Part model, mm, in its own coordinate system. Round coordinates to 2 decimals unless told otherwise and drop trailing zeros. Loops run counter-clockwise (first coordinate to the right, second up) from the corner with the lowest first, then second, coordinate; pieces in that order, holes last. Notation, with made-up numbers: (26.25, -40) - (70.25, -40) arc R28 cw to (70.25, -15) - close; hole circle Ø1 at (7, 27). An arc over 180 degrees is marked (long way). Write each question's results on one line, items separated by ' | '. Start each with the question number.
(1) Cut at B-B, the plane z = 5. List the corners of the cut face in (x, y), then the cut area to 3 significant figures.
(2) Mould opens along X. For faces 1 (the face through (0, 41, 0)), 2 (the face through (0.273, 42.282, 7.918)), 3 (the face through (-14.985, 42.479, 0.66)) say: released by +X, released by -X, zero draft, split by the parting line, or undercut.
(3) Cut at A-A, the plane x = 0. List the corners of the cut face in (y, z).
(4) Drill centre lines: L1, parallel to Z at x = 0, y = 42.8; L2, parallel to Z at x = 1.75, y = 41.75; L3, parallel to X at y = 43.9, z = 8. Where is each one in solid material? Low to high.
(5) Cut at C-C, the plane y = 41.7. List the corners of the cut face in (x, z), then the cut area to 3 significant figures.
(6) Cut at D-D, the plane z = -10. List the corners of the cut face in (x, y).
from build123d import *

# Parameters (mm, degrees)
SKETCH_1_R                  = 15
EXTRUDE_1_DEPTH             = 3
HOLE_WIZARD_M41_D           = 4.2
HOLE_WIZARD_M41_CSINK_D     = 5
HOLE_WIZARD_M41_CSINK_ANGLE = 90


with BuildPart() as part:
    # Эскиз1 → Бобышка-Вытянуть1 (new body)
    with BuildSketch(Plane.XZ.offset(-41)):
        Circle(SKETCH_1_R)
    extrude(amount=-EXTRUDE_1_DEPTH)

    # Сверло под метчик  спиральное M41 (through all)
    with Locations(Plane(origin=(0, 44, 0), x_dir=(1, 0, 0), z_dir=(0, 1, 0))):
        with Locations((-8.660254038, 5), (0, 10), (8.660254038, 5), (8.660254038, -5), (0, -10), (-8.660254038, -5)):
            CounterSinkHole(HOLE_WIZARD_M41_D / 2, HOLE_WIZARD_M41_CSINK_D / 2, counter_sink_angle=HOLE_WIZARD_M41_CSINK_ANGLE)


solid = part.part
A:
1) outline: (-14.14, 41) - (-10.76, 41) - (-10.76, 43.6) - (-11.16, 44) - (-14.14, 44) - close; (-6.56, 41) - (6.56, 41) - (6.56, 43.6) - (6.16, 44) - (-6.16, 44) - (-6.56, 43.6) - close; (10.76, 41) - (14.14, 41) - (14.14, 44) - (11.16, 44) - (10.76, 43.6) - close | area: 59.3 mm2
2) face 1: zero draft | face 2: undercut | face 3: split by the parting line
3) outline: (41, -15) - (44, -15) - (44, -12.5) - (43.6, -12.1) - (41, -12.1) - close; (41, -7.9) - (43.6, -7.9) - (44, -7.5) - (44, 7.5) - (43.6, 7.9) - (41, 7.9) - close; (41, 12.1) - (43.6, 12.1) - (44, 12.5) - (44, 15) - (41, 15) - close
4) L1: -15 to -12.1, -7.9 to 7.9, 12.1 to 15 | L2: -14.9 to -11.16, -8.84 to 8.84, 11.16 to 14.9 | L3: -12.69 to -1.33, 1.33 to 12.69
5) outline: circle Ø30 at (0, 0); hole circle Ø4.2 at (-8.66, -5); hole circle Ø4.2 at (-8.66, 5); hole circle Ø4.2 at (0, -10); hole circle Ø4.2 at (0, 10); hole circle Ø4.2 at (8.66, -5); hole circle Ø4.2 at (8.66, 5) | area: 624 mm2
6) outline: (-11.18, 41) - (-2.1, 41) - (-2.1, 43.6) - (-2.5, 44) - (-11.18, 44) - close; (2.1, 41) - (11.18, 41) - (11.18, 44) - (2.5, 44) - (2.1, 43.6) - close
